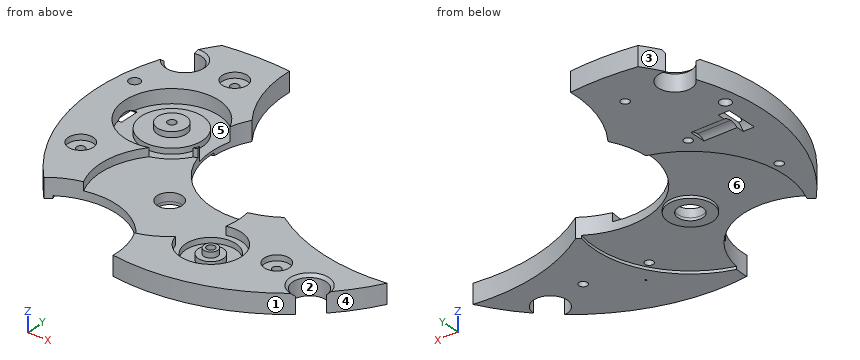
from build123d import *

# Parameters (mm, degrees)
CROQUIS2_R                 = 1.125
CROQUIS2_R_2               = 0.5
SALIENTE_EXTRUIR1_DEPTH    = 1.75
CORTAR_EXTRUIR1_DEPTH      = 0.75
CROQUIS4_R                 = 8.5
CORTAR_EXTRUIR2_DEPTH      = 0.25
CROQUIS5_R                 = 2.25
CROQUIS5_R_2               = 1.125
CORTAR_EXTRUIR3_DEPTH      = 0.5
CROQUIS6_R                 = 0.625
SALIENTE_EXTRUIR2_DEPTH    = 0.5
CROQUIS7_R                 = 4.25
CORTAR_EXTRUIR4_DEPTH      = 1.25
CROQUIS8_R                 = 2.75
SALIENTE_EXTRUIR3_DEPTH    = 0.5
CROQUIS9_R                 = 1.3
SALIENTE_EXTRUIR4_DEPTH    = 0.5
CROQUIS10_R                = 0.075
CORTAR_EXTRUIR5_DEPTH      = 1.5
CROQUIS11_R                = 1.125
CORTAR_EXTRUIR6_DEPTH      = 0.5
TALADRO_ROSCADO_M1X0_251_D = 0.75
TALADRO_ROSCADO_M1X0_253_D = 0.75
CHAFL_N1_SIZE              = 0.25
CROQUIS16_R                = 2
CROQUIS16_R_2              = 1.125
SALIENTE_EXTRUIR5_DEPTH    = 0.25
CROQUIS19_R                = 1.75
CORTAR_EXTRUIR7_DEPTH      = 1
CROQUIS20_R                = 1.25
CORTAR_EXTRUIR8_DEPTH      = 3
TALADRO_ROSCADO_M1X0_252_D = 0.75


with BuildPart() as part:
    # Croquis2 → Saliente-Extruir1 (new body)
    with BuildSketch(Plane.XY):
        with BuildLine():
            ThreePointArc((-16.326658805, 6.300016846), (-17.182882286, -3.316407146), (-12.80940905, -11.92346593))
            ThreePointArc((-12.80940905, -11.92346593), (-5.775317693, -11.220617232), (-2.259619844, -17.353504492))
            ThreePointArc((-2.259619844, -17.353504492), (4.841189817, -16.817041391), (11.1403887, -13.49598976))
            ThreePointArc((11.1403887, -13.49598976), (10.224088307, -10.905694194), (12.74994394, -11.987031723))
            ThreePointArc((12.74994394, -11.987031723), (14.176723516, -10.260141829), (15.371220143, -8.365141441))
            ThreePointArc((15.371220143, -8.365141441), (9.460159173, -8.065624613), (4.022288522, -5.728978535))
            ThreePointArc((4.022288522, -5.728978535), (-4.686054245, -5.200086116), (-6.115237098, 3.406446129))
            ThreePointArc((-6.115237098, 3.406446129), (-7.762325395, 6.723591586), (-8.243034525, 10.395821504))
            ThreePointArc((-8.243034525, 10.395821504), (-11.230553814, 10.48910556), (-14.20719972, 10.21789979))
            ThreePointArc((-14.20719972, 10.21789979), (-14.787393079, 9.358579269), (-15.315676961, 8.466406511))
            ThreePointArc((-15.315676961, 8.466406511), (-13.64072529, 6.365671802), (-16.326658805, 6.300016846))
        make_face()
        with Locations((-4.5875, -7.94578308)):
            Circle(CROQUIS2_R, mode=Mode.SUBTRACT)
        with Locations((-16, 2.5)):
            Circle(CROQUIS2_R_2, mode=Mode.SUBTRACT)
    extrude(amount=SALIENTE_EXTRUIR1_DEPTH)

    # Croquis3 → Cortar-Extruir1 (cut)
    with BuildSketch(Plane.XY.offset(1.75)):
        with BuildLine():
            ThreePointArc((1.526213137, -9.243863075), (-10.000158774, -4.82078308), (-0.406473179, -12.59137397))
            ThreePointArc((-0.406473179, -12.59137397), (4.63567055, -13.27078308), (1.526213137, -9.243863075))
        make_face()
    extrude(amount=-CORTAR_EXTRUIR1_DEPTH, mode=Mode.SUBTRACT)

    # Croquis4 → Cortar-Extruir2 (cut)
    with BuildSketch(Plane(origin=(0, 0, 0), x_dir=(-1, 0, 0), z_dir=(0, 0, -1))):
        with Locations((4.5875, -7.94578308)):
            Circle(CROQUIS4_R)
    extrude(amount=-CORTAR_EXTRUIR2_DEPTH, mode=Mode.SUBTRACT)

    # Croquis5 → Cortar-Extruir3 (cut)
    with BuildSketch(Plane.XY.offset(1)):
        with Locations((2.25410069, -11.89578308)):
            Circle(CROQUIS5_R)
        with Locations((2.25410069, -11.89578308)):
            Circle(CROQUIS5_R_2, mode=Mode.SUBTRACT)
    extrude(amount=-CORTAR_EXTRUIR3_DEPTH, mode=Mode.SUBTRACT)

    # Croquis6 → Saliente-Extruir2 (add)
    with BuildSketch(Plane.XY.offset(1)):
        with Locations((2.25410069, -11.89578308)):
            Circle(CROQUIS6_R)
    extrude(amount=SALIENTE_EXTRUIR2_DEPTH)

    # Croquis7 → Cortar-Extruir4 (cut)
    with BuildSketch(Plane.XY.offset(1.75)):
        with Locations((-10.659116856, 0)):
            Circle(CROQUIS7_R)
    extrude(amount=-CORTAR_EXTRUIR4_DEPTH, mode=Mode.SUBTRACT)

    # Croquis8 → Saliente-Extruir3 (add)
    with BuildSketch(Plane.XY.offset(0.5)):
        with Locations((-10.659116856, 0)):
            Circle(CROQUIS8_R)
    extrude(amount=SALIENTE_EXTRUIR3_DEPTH)

    # Croquis9 → Saliente-Extruir4 (add)
    with BuildSketch(Plane.XY.offset(1)):
        with Locations((-10.659116856, 0)):
            Circle(CROQUIS9_R)
    extrude(amount=SALIENTE_EXTRUIR4_DEPTH)

    # Croquis10 → Cortar-Extruir5 (cut, through all)
    with BuildSketch(Plane.XY.offset(0.5)):
        with Locations((3.668314252, -13.309996642)):
            Circle(CROQUIS10_R)
    extrude(amount=-CORTAR_EXTRUIR5_DEPTH, mode=Mode.SUBTRACT)

    # Croquis11 → Cortar-Extruir6 (cut)
    with BuildSketch(Plane.XY.offset(1.75)):
        with Locations((-13.75, -6.5)):
            Circle(CROQUIS11_R)
        with Locations((-10.5, 7)):
            Circle(CROQUIS11_R)
        with Locations((7.5, -11)):
            Circle(CROQUIS11_R)
    extrude(amount=-CORTAR_EXTRUIR6_DEPTH, mode=Mode.SUBTRACT)

    # Taladro roscado M1x0.251 (through all)
    with Locations(Plane.XY.offset(1.5)):
        with Locations((2.25410069, -11.89578308)):
            Hole(TALADRO_ROSCADO_M1X0_251_D / 2)

    # Taladro roscado M1x0.253 (through all)
    with Locations(Plane.XY.offset(1.5)):
        with Locations((-10.659116856, 0)):
            Hole(TALADRO_ROSCADO_M1X0_253_D / 2)

    # Chaflán1
    chafl_n1_edges = [part.edges().sort_by_distance(p)[0] for p in [
        (10.224088307, -10.905694194, 1.75),
        (-13.64072529, 6.365671802, 1.75),
    ]]
    chamfer(chafl_n1_edges, length=CHAFL_N1_SIZE)

    # Croquis16 → Saliente-Extruir5 (add)
    with BuildSketch(Plane(origin=(0, 0, 0.25), x_dir=(-1, 0, 0), z_dir=(0, 0, -1))):
        with Locations((4.5875, -7.94578308)):
            Circle(CROQUIS16_R)
        with Locations((4.5875, -7.94578308)):
            Circle(CROQUIS16_R_2, mode=Mode.SUBTRACT)
    extrude(amount=SALIENTE_EXTRUIR5_DEPTH)

    # Croquis19 → Cortar-Extruir7 (cut)
    with BuildSketch(Plane(origin=(-14.5, 0, 0), x_dir=(0, 0, -1), z_dir=(1, 0, 0))):
        with Locations((1, 0)):
            Circle(CROQUIS19_R)
    extrude(amount=-CORTAR_EXTRUIR7_DEPTH, mode=Mode.SUBTRACT)

    # Croquis20 → Cortar-Extruir8 (cut)
    with BuildSketch(Plane.ZY.offset(14.5)):
        with Locations((-1, 0)):
            Circle(CROQUIS20_R)
    extrude(amount=-CORTAR_EXTRUIR8_DEPTH, mode=Mode.SUBTRACT)

    # Taladro roscado M1x0.252 (through all)
    with Locations(Plane.XY.offset(1.25)):
        with Locations((-13.75, -6.5), (-10.5, 7), (7.5, -11)):
            Hole(TALADRO_ROSCADO_M1X0_252_D / 2)


solid = part.part
Verification items for the finished model (mm, model axes). Face numbers are marked on the shaded views. A direction names the side the tool comes from. Coordinates: 2 decimals unless noted, no trailing zeros. Loops run counter-clockwise (first coordinate to the right, second up) from the corner with the lowest first, then second, coordinate; pieces in that order, holes last. Notation, with made-up numbers: (74.5, -29) -> (83.5, -29) arc R11 cw to (83.5, -20) -> close; hole circle Ø6 at (34, 3). An arc over 180 degrees is marked (long way). Answer as CSV lines item,"result".
1) Cross-section at C-C, the plane y = -3.5. Record the cut outline in (x, z), then the cut area to 3 significant figures.
Found:
outline,"(-17.15, 0) -> (-11.83, 0) -> (-11.83, 0.25) -> (-6.06, 0.25) -> (-6.06, 1) -> (-8.25, 1) -> (-8.25, 0.5) -> (-13.07, 0.5) -> (-13.07, 1.75) -> (-17.15, 1.75) -> close"
area,"10.3 mm2"
2) Thickness scan on L1, parallel to Y at x = -10.5, z = 0.8 (3 decimals); L2, parallel to X at y = -11.25, z = 0.55; L3, parallel to X at y = -14.25, z = 1.55. Record the ranges inside material, lowest first. Write a range as from..to.
Found:
L1,"y = -10.74..-4.247, -2.745..-0.34, 0.34..2.745, 4.247..6.625, 7.375..10.5"
L2,"x = -13.4..-11.78, -5.72..0.1, 1.33..3.18, 4.41..7.22, 7.78..9.95, 12.55..13.4"
L3,"x = -2.86..0.83, 3.68..10.16"
3) Release check for a two-part mould opening along X. For the marked faces 1, 2 and 3 record: +X half, -X half, draft (parallel to the pull), parting line (faces both ways), or undercut.
Found:
face 1,"parting line"
face 2,"undercut"
face 3,"-X half"
4) Cross-section at B-B, the plane y = 7. Record the cut outline in (x, z) (3 decimals).
Found:
outline,"(-13.5, 0) -> (-10.875, 0) -> (-10.875, 1.25) -> (-11.625, 1.25) -> (-11.625, 1.75) -> (-13.25, 1.75) -> (-13.5, 1.5) -> close; (-10.125, 0) -> (-7.843, 0) -> (-7.843, 1.75) -> (-9.375, 1.75) -> (-9.375, 1.25) -> (-10.125, 1.25) -> close"
5) Cross-section at D-D, the plane x = -4.5. Record the cut outline in (y, z), then the cut area to 3 significant figures.
Found:
outline,"(-12.08, 0.25) -> (-9.94, 0.25) -> (-9.94, 0) -> (-9.07, 0) -> (-9.07, 1) -> (-12.08, 1) -> close; (-6.82, 0) -> (-5.95, 0) -> (-5.95, 0.25) -> (-5.36, 0.25) -> (-5.36, 1) -> (-6.82, 1) -> close"
area,"3.80 mm2"
6) Depth check by flat-ended pin: pin 1 (3.5 mm diameter, centred on x = -4.59, y = -7.95, fed in from -Z); pin 2 (3 mm diameter, centred on x = -11, y = 1, fed in from +Z); pin 3 (2 mm diameter, centred on x = -13.75, y = -6.5, fed in from +Z); pin 4 (1 mm diameter, centred on x = 1, y = -8.5, fed in from -Z). Enter the tip coordinate at first touch or a pass-through.
Found:
pin 1,"stops at z = 0"
pin 2,"stops at z = 1.5"
pin 3,"stops at z = 1.25"
pin 4,"stops at z = 0.25"
7) Tool access check on the marked faces 4, 5 and 6. Record the directions out of +Z, -Z, +X, -X, +Y, -Y that give a thin tool (end or side, any length) a straight path to the whole face; none if there is none.
Found:
face 4,"+Z, -Z, +X, -Y"
face 5,"+Z"
face 6,"-Z"
8) Cross-section at A-A, the plane x = 7.5. Record the cut outline in (y, z) (3 decimals), then the cut area to 3 significant figures.
Found:
outline,"(-15.811, 0) -> (-11.375, 0) -> (-11.375, 1.25) -> (-12.125, 1.25) -> (-12.125, 1.75) -> (-15.811, 1.75) -> close; (-10.625, 0) -> (-7.482, 0) -> (-7.482, 1.75) -> (-9.875, 1.75) -> (-9.875, 1.25) -> (-10.625, 1.25) -> close"
area,"12.5 mm2"
